The drawing under review shows one solid part. Ordinate dimensions are in mm from its lowest x, y, z. Round coordinates to 2 decimals unless told otherwise and drop trailing zeros. Write each loop counter-clockwise with the first axis right and the second up, starting at its lowest first coordinate (ties: lowest second). Pieces come first, ordered by that corner, then holes. Notation, with made-up numbers: M -33.75,73 L 8.25,73 A19 cw 8.25,83 Z; hole C 26.25,-9 d11. An arc over 180 degrees is marked long. Write item = value, one per line. Start each with the question number.
Item 1: Take a section at C-C, the plane x = 55. Give the boundary of the cut face in (y, z).
Item 2: Take a section at A-A, the plane z = 1.2. Give the boundary of the cut face in (x, y).
Item 3: Take a section at B-B, the plane y = 7.5. Give the boundary of the cut face in (x, z).
Item 4: For pin 1 Ø1.9 at (x, y) = (5, 7.5) entering from -Z, flat-tipped, find the tip position at first contact; note if it passes through.
Item 5: Take a section at D-D, the plane x = 10.5. Give the boundary of the cut face in (y, z), plus the area to 3 significant figures.
Item 6: To check wall thickness, follow line 1 along X through (y, z) = (7.5, 0.6); line 2 along Y through (x, z) = (55, 1.5) (1 decimal); line 3 along Y through (x, z) = (30.5, 1.75). State the ranges of each line that lie inside material, in increasing order.
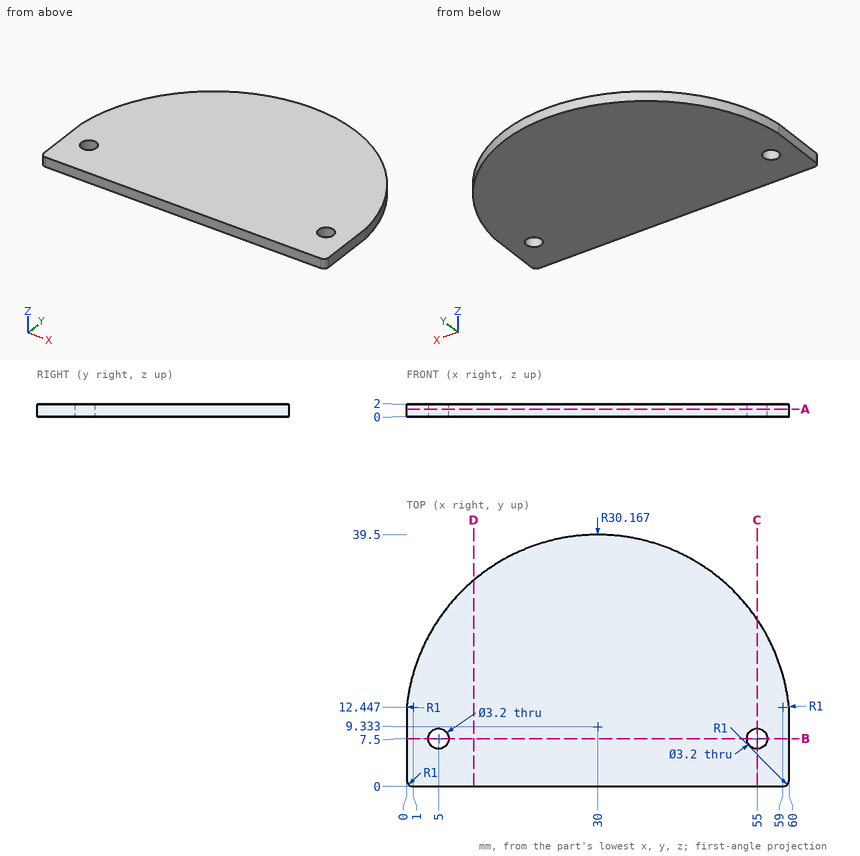
Response values:
q1.outline = M 0,0 L 5.9,0 L 5.9,2 L 0,2 Z; M 9.1,0 L 26.22,0 L 26.22,2 L 9.1,2 Z
q2.outline = M 0,1 A1 ccw 1,0 L 59,0 A1 ccw 60,1 L 60,12.45 A1 ccw 59.99,12.55 A30.17 ccw 0.01,12.55 A1 ccw 0,12.45 Z; hole C 5,7.5 d3.2; hole C 55,7.5 d3.2
q3.outline = M 0,0 L 3.4,0 L 3.4,2 L 0,2 Z; M 6.6,0 L 53.4,0 L 53.4,2 L 6.6,2 Z; M 56.6,0 L 60,0 L 60,2 L 56.6,2 Z
q4.pin_1 = through
q5.outline = M 0,0 L 32.35,0 L 32.35,2 L 0,2 Z
q5.area = 64.7 mm2
q6.line_1 = 0 to 3.4, 6.6 to 53.4, 56.6 to 60
q6.line_2 = 0 to 5.9, 9.1 to 26.2
q6.line_3 = 0 to 39.5
